from build123d import *

# Parameters (mm, degrees)
SKETCH1_W           = 28
SKETCH1_H           = 22.2
SKETCH1_R           = 1.5
BOSS_EXTRUDE1_DEPTH = 1
SKETCH2_W           = 7.140567323
SKETCH2_H           = 10.37472735
SKETCH2_W_2         = 7.324889891
SKETCH2_H_2         = 10.322063759
SKETCH2_W_3         = 2.374512373
SKETCH2_H_3         = 15.114450504
BOSS_EXTRUDE2_DEPTH = 6.5


with BuildPart() as part:
    # Sketch1 → Boss-Extrude1 (new body)
    with BuildSketch(Plane(origin=(0, 0, 0), x_dir=(1, 0, 0), z_dir=(0, 1, 0))):
        with Locations((14, 11.1)):
            Rectangle(SKETCH1_W, SKETCH1_H)
        with Locations((9.4, 20)):
            Circle(SKETCH1_R, mode=Mode.SUBTRACT)
        with Locations((22.4, 20)):
            Circle(SKETCH1_R, mode=Mode.SUBTRACT)
        with Locations((22.4, 2.2)):
            Circle(SKETCH1_R, mode=Mode.SUBTRACT)
        with Locations((9.4, 2.2)):
            Circle(SKETCH1_R, mode=Mode.SUBTRACT)
    extrude(amount=BOSS_EXTRUDE1_DEPTH)

    # Sketch2 → Boss-Extrude2 (add)
    with BuildSketch(Plane.XZ):
        with Locations((3.570283662, -16.616511116)):
            Rectangle(SKETCH2_W, SKETCH2_H)
        with Locations((3.662444946, -5.399166316)):
            Rectangle(SKETCH2_W_2, SKETCH2_H_2)
        with Locations((26.812743813, -10.797184354)):
            Rectangle(SKETCH2_W_3, SKETCH2_H_3)
    extrude(amount=BOSS_EXTRUDE2_DEPTH)


solid = part.part
The listing builds one solid part. Answer for the finished solid, in the listing's coordinates (mm). A direction names the side the tool comes from. Coordinates: 2 decimals unless noted, no trailing zeros. Order: outer loops, then holes, each group sorted by start corner. A loop starts at its lowest first (then second) coordinate and runs counter-clockwise, first axis right, second up. Notation, with made-up numbers: (-17.5, 47) -> (40.5, 47) arc R19 ccw to (40.5, 81) -> close; hole circle Ø8 at (-0.5, -11). An arc over 180 degrees is marked (long way). Answer in a Markdown table with one row per item. Add a question column.
Item 1: Which of the six approach directions +Z, -Z, +X, -X, +Y, -Y give full straight-line access (tool end or side, diameter ignored) to faces 1 (the face through (4, -6.5, -5)), 2 (the face through (4, -3, -0.238)), 3 (the face through (7.325, -3, -5)), 4 (the face through (4, -3, -10.56)), 5 (the face through (4, -3, -21.804))?
Item 2: Find section B-B (y = -4). Write down the section's boundary in (x, z), then the cut area to 3 significant figures.
Item 3: Determine the mould class of faces 6 (the face through (0, -3, -13)), 7 (the face through (27, -3, -18.354)), 8 (the face through (14, 0, -11)) for opening direction X: +X half, -X half, draft (parallel to the pull), parting line (faces both ways), or undercut.
Item 4: Find section C-C (x = 9.4). Write down the section's boundary in (y, z).
Item 5: Find section D-D (z = -5.5). Write down the section's boundary in (x, y).
Item 6: Each of these flat-tipped pins is pushed along its axis until it touches: P1, Ø2, axis at x = 24, y = -5.5, coming from the -Z side; P2, Ø1.9, axis at x = 27.5, y = -3, coming from the -Z side; P3, Ø1.9, axis at x = 26.5, y = -2.5, coming from the +Z side; P4, Ø2, axis at x = 3, y = -1.5, coming from the -Z side. Where does it stop, or does it pass through?
Item 7: Find section A-A (z = -2.2). Write down the section's boundary in (x, y).
Item 8: Find the intervals of material crossed by L1, parallel to Z at x = 9.4, y = 0.6; L2, parallel to X at y = 0.7, z = -20; L3, parallel to X at y = -2.5, z = -17, in increasing order. Write a range as from..to.
Result set:
| question | item | result |
|---|---|---|
| 1 | face 1 | +Z, -Z, +X, -X, -Y |
| 1 | face 2 | +Z, +X, -X, -Y |
| 1 | face 3 | +Z, -Z, -Y |
| 1 | face 4 | -X, -Y |
| 1 | face 5 | -Z, +X, -X, -Y |
| 2 | outline | (0, -21.8) -> (7.14, -21.8) -> (7.14, -11.43) -> (0, -11.43) -> close; (0, -10.56) -> (7.32, -10.56) -> (7.32, -0.24) -> (0, -0.24) -> close; (25.63, -18.35) -> (28, -18.35) -> (28, -3.24) -> (25.63, -3.24) -> close |
| 2 | area | 186 mm² |
| 3 | face 6 | -X half |
| 3 | face 7 | draft |
| 3 | face 8 | undercut |
| 4 | outline | (0, -22.2) -> (1, -22.2) -> (1, -21.5) -> (0, -21.5) -> close; (0, -18.5) -> (1, -18.5) -> (1, -3.7) -> (0, -3.7) -> close; (0, -0.7) -> (1, -0.7) -> (1, 0) -> (0, 0) -> close |
| 5 | outline | (0, -6.5) -> (7.32, -6.5) -> (7.32, 0) -> (25.63, 0) -> (25.63, -6.5) -> (28, -6.5) -> (28, 1) -> (0, 1) -> close |
| 6 | P1 | passes through |
| 6 | P2 | stops at z = -18.35 |
| 6 | P3 | stops at z = -3.24 |
| 6 | P4 | stops at z = -21.8 |
| 7 | outline | (0, -6.5) -> (7.32, -6.5) -> (7.32, 0) -> (7.9, 0) -> (7.9, 1) -> (0, 1) -> close; (10.9, 0) -> (20.9, 0) -> (20.9, 1) -> (10.9, 1) -> close; (23.9, 0) -> (28, 0) -> (28, 1) -> (23.9, 1) -> close |
| 8 | L1 | z = -22.2..-21.5, -18.5..-3.7, -0.7..0 |
| 8 | L2 | x = 0..7.9, 10.9..20.9, 23.9..28 |
| 8 | L3 | x = 0..7.14, 25.63..28 |
